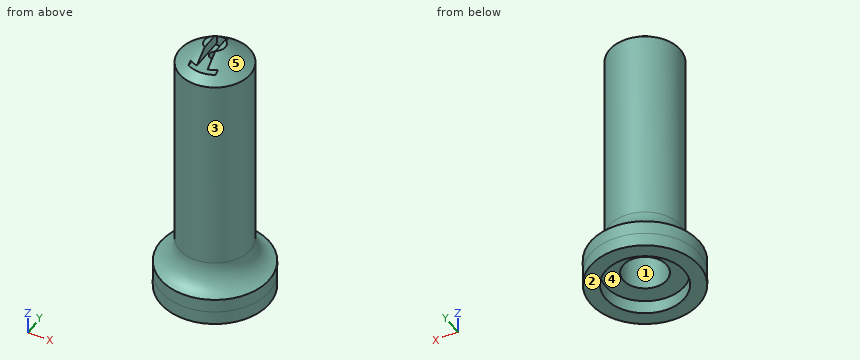
```python
from build123d import *

# Parameters (mm, degrees)
F0_W     = 2.5
F0_H     = 2.5
F0_W_2   = 3.5
F3_W     = 1.9934664722
F3_H     = 2
F3_H_2   = 0.5
F3_W_2   = 1.5032667639
F4_DEPTH = 27.5
F5_R     = 10
F5_R_2   = 7.25
F6_DEPTH = 2.5


# Not quite as in the source:
# - a fillet or chamfer that OpenCascade refuses, or shapes differently, is made with other operations: its cross-section is extruded or revolved along the edge and cut away or added


with BuildPart() as f1:
    # F0 (on Front) → F1 (revolve)
    with BuildSketch(Plane.XZ):
        Polygon((-6.5, 0), (-4, 0), (-4, 40), (-1, 42.5), (0, 42.5), (0, 45), (-1.905124838, 45), (-6.5, 41.170937365), align=None)
        with Locations((-5.25, -1.25)):
            Rectangle(F0_W, F0_H)
        with Locations((-8.25, -1.25)):
            Rectangle(F0_W_2, F0_H)
    revolve(axis=Axis((0, 0, 20), (0, 0, 1)))

    # F3 (on offset) → F4 (cut)
    with BuildSketch(Plane.XZ.offset(25)):
        with Locations((0, 44)):
            Rectangle(F3_W, F3_H)
        with Locations((0, 42.75)):
            Rectangle(F3_W, F3_H_2)
        with Locations((-1.7483666181, 42.75)):
            Rectangle(F3_W_2, F3_H_2)
        with Locations((1.7483666181, 42.75)):
            Rectangle(F3_W_2, F3_H_2)
    extrude(amount=-F4_DEPTH, mode=Mode.SUBTRACT)

    # F5 (on face) → F6 (join)
    with BuildSketch(Plane(origin=(0, 0, -2.5), x_dir=(1, 0, 0), z_dir=(0, 0, -1))):
        Circle(F5_R)
        Circle(F5_R_2, mode=Mode.SUBTRACT)
    extrude(amount=F6_DEPTH)

    # F7: fillet of radius 5 on 1 edges, made by hand

    # F7_s1 → F7_t2 (revolve)
    with BuildSketch(Plane.XZ):
        with BuildLine():
            ThreePointArc((-6.5, 4.7696960071), (-7.4688711259, 1.8116561155), (-10, 0))
            Line((-10, 0), (-6.5, 0))
            Line((-6.5, 0), (-6.5, 4.7696960071))
        make_face()
    revolve(axis=Axis((0, 0, 0), (0, 0, 1)))


solid = f1.part
```
Can you work these out from the model? Positions are in its coordinate system, mm. Face numbers are marked on the shaded views. A direction names the side the tool comes from. Give positions to 0.01 mm unless a question says otherwise; leave off trailing zeros. Write each loop counter-clockwise with the first axis right and the second up, starting at its lowest first coordinate (ties: lowest second). Pieces come first, ordered by that corner, then holes. Notation, with made-up numbers: (4.25, -40) -> (18.25, -40) arc R17 cw to (18.25, -12) -> close; hole circle Ø3 at (19, 78). An arc over 180 degrees is marked (long way). Write item = value, one per line.
(1) I'm going to push flat-ended pins straight in: P1, Ø0.5, axis at x = -2, y = -0.5, coming from the -Z side; P2, Ø1.6, axis at y = -1, z = 44, coming from the +X side; P3, Ø1.5, axis at x = 0.5, y = 5.5, coming from the +Z side. Where does each tip first touch, or does it pass through?
Worked out:
P1 = 41.41
P2 = 3.96
P3 = 42.61
(2) Suppose I cut it at B-B on y = 0. Write out the boundary of the cut face in (x, z), then the cut area to 3 significant figures.
Worked out:
outline = (-10, -5) -> (-7.25, -5) -> (-7.25, -2.5) -> (-4, -2.5) -> (-4, 40) -> (-1, 42.5) -> (-2.5, 42.5) -> (-2.5, 43) -> (-1, 43) -> (-1, 45) -> (-1.91, 45) -> (-6.5, 41.17) -> (-6.5, 4.77) arc R5 cw to (-10, 0) -> close; (1, 42.5) -> (4, 40) -> (4, -2.5) -> (7.25, -2.5) -> (7.25, -5) -> (10, -5) -> (10, 0) arc R5 cw to (6.5, 4.77) -> (6.5, 41.17) -> (1.91, 45) -> (1, 45) -> (1, 43) -> (2.5, 43) -> (2.5, 42.5) -> close
area = 281 mm^2
(3) I need wall thicknesses on probe 1 along Y at (x, z) = (0, 10); probe 2 along X at (y, z) = (0, -3.9). Which ranges of each line are inside material? Lowest first, please. Write a range as from..to.
Worked out:
probe_1 = -6.5..-4, 4..6.5
probe_2 = -10..-7.25, 7.25..10
(4) Thinking about a two-plate mould opening in X: for the marked faces 1, 2 and 3, which applies, released by +X, released by -X, zero draft, split by the parting line, or undercut?
Worked out:
face_1 = undercut
face_2 = zero draft
face_3 = split by the parting line
(5) Suppose I cut it at C-C on z = 26. Write out the boundary of the cut face in (x, y).
Worked out:
outline = circle Ø13 at (0, 0); hole circle Ø8 at (0, 0)
(6) Suppose I cut it at A-A on x = 0. Write out the boundary of the cut face in (y, z).
Worked out:
outline = (-10, -5) -> (-7.25, -5) -> (-7.25, -2.5) -> (-4, -2.5) -> (-4, 40) -> (-1, 42.5) -> (-4.91, 42.5) -> (-6.5, 41.17) -> (-6.5, 4.77) arc R5 cw to (-10, 0) -> close; (1, 42.5) -> (4, 40) -> (4, -2.5) -> (7.25, -2.5) -> (7.25, -5) -> (10, -5) -> (10, 0) arc R5 cw to (6.5, 4.77) -> (6.5, 41.17) -> (2.5, 44.5) -> (2.5, 42.5) -> close
(7) For the marked faces 4 and 5, which set-ups out of +Z, -Z, +X, -X, +Y, -Y let a thin tool reach every point of the face, with its end or its side?
Worked out:
face_4 = -Z
face_5 = +Z
